Source: CAD feature listing. Evaluate the final solid. Frame: model axes, mm. A direction names the side the tool comes from. Give positions to 0.01 mm unless a question says otherwise; leave off trailing zeros. Loops run counter-clockwise (first coordinate to the right, second up) from the corner with the lowest first, then second, coordinate; pieces in that order, holes last. Notation, with made-up numbers: (-9, 30) -> (27, 30) arc R17 ccw to (27, 44) -> close; hole circle Ø3 at (62.5, -32). An arc over 180 degrees is marked (long way). Return JSON: item names as keys, results as strings. Group by question number.
```python
from build123d import *

# Parameters (mm, degrees)
F1_DEPTH = 596.9
F2_R     = 5.08
F3_R     = 7.14375
F4_DEPTH = 25.4


with BuildPart() as f1:
    # F0 (on Front) → F1 (new body, symmetric)
    with BuildSketch(Plane.XZ):
        Polygon((-38.1, -38.1), (38.1, -38.1), (38.1, -31.75), (-31.75, -31.75), (-31.75, 38.1), (-38.1, 38.1), align=None)
    extrude(amount=F1_DEPTH, both=True)

    # F2
    f2_edges = [f1.edges().sort_by_distance(p)[0] for p in [
        (-31.75, 0, 38.1),
        (-31.75, 0, -31.75),
        (38.1, 0, -31.75),
    ]]
    fillet(f2_edges, radius=F2_R)

    # F3 (on face) → F4 (cut)
    with BuildSketch(Plane(origin=(0, 0, -38.1), x_dir=(1, 0, 0), z_dir=(0, 0, -1))):
        with Locations((6.35, -565.15)):
            Circle(F3_R)
    extrude(amount=-F4_DEPTH, mode=Mode.SUBTRACT)


solid = f1.part
```
1) Material intervals for line 1 (Y direction, x = 6.35, z = -34); line 2 (X direction, y = 408, z = -17), sorted ascending.
2) Mould query, pull axis X, two halves, no side actions, for faces 3 (the face through (-31.75, -8, 3)), 4 (the face through (-38.1, -8, 1)), 5 (the face through (-34, 596.9, -14)). Classes: released by +X, released by -X, zero draft, split by the parting line, or undercut.
3) Reachability of faces 1 (the face through (4, -8, -31.75)), 2 (the face through (-1, -8, -38.1)) from +Z, -Z, +X, -X, +Y, -Y: full face, straight path, thin tool, end or side. Return the list, or none.
4) Cut plane A-A on y = 227.5. Return loops of the section in (x, z).
5) Cut plane B-B on z = -14. Return loops of the section in (x, y).
Calculated:
{
 "1": {"line 1": "-596.9 to 558.01, 572.29 to 596.9", "line 2": "-38.1 to -31.75"},
 "2": {"face 3": "released by +X", "face 4": "released by -X", "face 5": "zero draft"},
 "3": {"face 1": "+Z, +X, +Y, -Y", "face 2": "-Z, +X, -X, +Y, -Y"},
 "4": {"outline": "(-38.1, -38.1) -> (38.1, -38.1) -> (38.1, -36.83) arc R5.08 ccw to (33.02, -31.75) -> (-26.67, -31.75) arc R5.08 cw to (-31.75, -26.67) -> (-31.75, 33.02) arc R5.08 ccw to (-36.83, 38.1) -> (-38.1, 38.1) -> close"},
 "5": {"outline": "(-38.1, -596.9) -> (-31.75, -596.9) -> (-31.75, 596.9) -> (-38.1, 596.9) -> close"}
}
